Could you check a few things on this model? Use its own coordinates, in mm. Face numbers are marked on the shaded views. A direction names the side the tool comes from. Round coordinates to 2 decimals unless told otherwise and drop trailing zeros. Loops run counter-clockwise (first coordinate to the right, second up) from the corner with the lowest first, then second, coordinate; pieces in that order, holes last. Notation, with made-up numbers: M 16.5,54 L 49.5,54 A15 cw 49.5,63 Z; hole C 1.5,-30.5 d8. An arc over 180 degrees is marked long. Answer in a Markdown table with one row per item.
Autodesk Inventor part; units mm, degrees
ref_plane "YZ Plane" through (0, 0, 0) normal (1, 0, 0) x (0, 1, 0)
ref_plane "XZ Plane" through (0, 0, 0) normal (0, 1, 0) x (-1, 0, 0)
ref_plane "XY Plane" through (0, 0, 0) normal (0, 0, 1) x (1, 0, 0)
sketch "Sketch1" plane through (0, 0, 0) normal (0, 0, 1) x (1, 0, 0)
  line L0 (0, 0) -> (35, 0)
  line L1 (35, 0) -> (35, 82)
  line L2 (35, 82) -> (0, 82)
  line L3 (0, 82) -> (0, 0)
  line L4 (8.5, 79.95) -> (8.5, 77.05)
  line L5 (8.5, 77.05) -> (5.5, 77.05)
  line L6 (5.5, 77.05) -> (5.5, 53.95)
  line L7 (5.5, 33.6) -> (5.5, 6.85)
  line L8 (5.5, 6.85) -> (29.5, 6.85)
  line L9 (29.5, 6.85) -> (29.5, 79.95)
  line L10 (29.5, 79.95) -> (8.5, 79.95)
  line L11 (5.5, 53.95) -> (8.5, 53.95)
  line L12 (8.5, 53.95) -> (8.5, 33.6)
  line L13 (8.5, 33.6) -> (5.5, 33.6)
  circle A0 centre (19, 65.65) radius 2.25
  circle A1 centre (19, 21.45) radius 2.25
  dimension "d0" = 35
  dimension "d1" = 82
  dimension "d2" = 21
  dimension "d3" = 24
  dimension "d4" = 21
  dimension "d5" = 26.75
  dimension "d6" = 23.1
  dimension "d7" = 26
  dimension "d8" = 6.85
  dimension "d9" = 5.5
  dimension "d10" = 20.35
  dimension "d15" = 4.5
  dimension "d16" = 4.5
  dimension "d17" = 44.2
  dimension "d18" = 10.5
  dimension "d19" = 14.3
  dimension "d20" = 10.5
extrude "Extrusion1" add sketch "Sketch1" against normal blind 1.5 contours L10 L9 L8 L7 L13 L12 L11 L6 L5 L4 | A0 | A1
extrude "Extrusion3" add sketch "Sketch1" along normal blind 5 contours L3 L2 L1 L0 | L10 L9 L8 L7 L13 L12 L11 L6 L5 L4
sketch "Sketch2" plane through (0, 0, 5) normal (0, 0, 1) x (1, 0, 0)
  circle A0 centre (19, 21.45) radius 4.25
  circle A1 centre (19, 65.65) radius 4.25
  point P0 (0, 0)
  dimension "d23" = 8.5
  dimension "d24" = 8.5
extrude "Extrusion4" cut sketch "Sketch2" against normal blind 3
sketch "Sketch3" plane through (0, 0, 0) normal (0, -1, 0) x (1, 0, 0)
  line L0 (0, 5) -> (35, 5)
  line L1 (0, 0) -> (0, 5)
  line L2 (35, 0) -> (35, 5)
  line L3 (0, 5) -> (35, 5)
  line L4 (35, 5) -> (35, -32)
  line L5 (35, -32) -> (0, -32)
  line L6 (0, -32) -> (0, 5)
  line L7 (0, 0) -> (35, 0)
  line L8 (5.5, 0) -> (5.5, -1.5)
  line L9 (5.5, -8.5) -> (24.15, -8.5)
  line L10 (24.15, -8.5) -> (24.15, -11.35)
  line L11 (24.15, -11.35) -> (5.5, -11.35)
  line L12 (5.5, -11.35) -> (5.5, -8.5)
  dimension "d27" = 32
  dimension "d28" = 8.5
  dimension "d29" = 2.85
  dimension "d30" = 18.65
extrude "Extrusion5" add sketch "Sketch3" along normal blind 5 contours L0 L2 L7 L1 | L7 L4 L5 L6 | L9 L10 L11 L12
extrude "Extrusion6" add sketch "Sketch3" against normal blind 1.5 contours L9 L10 L11 L12
fillet "Fillet1" radius 1 1 edges at (29.5, 79.95, -0.75)
fillet "Fillet2" radius 1 1 edges at (8.5, 79.95, -0.75)
fillet "Fillet3" radius 1 1 edges at (5.5, 77.05, -0.75)
fillet "Fillet4" radius 1 1 edges at (5.5, 53.95, -0.75)
fillet "Fillet5" radius 1 1 edges at (5.5, 33.6, -0.75)
fillet "Fillet6" radius 1 1 edges at (5.5, 6.85, -0.75)
fillet "Fillet7" radius 1 1 edges at (29.5, 6.85, -0.75)
fillet "Fillet8" radius 1 1 edges at (5.5, 0.75, -11.35)
fillet "Fillet9" radius 1 3 edges at (24.15, 0.75, -11.35) (24.15, 0.75, -8.5) (5.5, 0.75, -8.5)
extrude "Extrusion7" cut sketch "Sketch1" against normal up to next contours A0 | A1
sketch "Sketch4" plane through (0, -5, 0) normal (0, -1, 0) x (1, 0, 0)
  line L0 (25.5, -24) -> (9.5, -24)
  line L1 (9.5, -24) -> (9.5, -8)
  line L2 (9.5, -8) -> (25.5, -8)
  line L3 (25.5, -8) -> (25.5, -24)
  line L4 (0, 5) -> (0, -32)
  line L5 (0, -32) -> (35, -32)
  point P0 (0, 0)
  dimension "d46" = 16
  dimension "d47" = 16
  dimension "d48" = 9.5
  dimension "d49" = 8
extrude "Extrusion8" add sketch "Sketch4" along normal blind 5
chamfer "Chamfer1" distance 5 angle 45 4 edges at (9.5, -5, -16) (17.5, -5, -24) (25.5, -5, -16) (17.5, -5, -8)
properties part number "keithley_2000_front_feet"
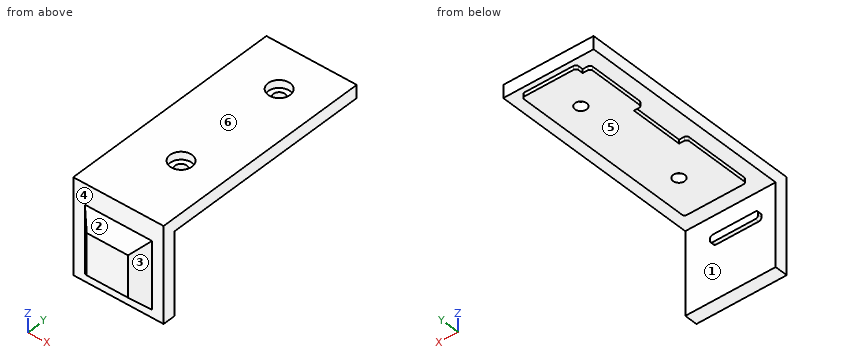
1) I want a section at D-D, the plane y = 47.5. Please give me the cut outline in (x, z), plus the area to 4 significant figures.
Computed:
| item | result |
|---|---|
| outline | M 0,0 L 8.5,0 L 8.5,-1.5 L 29.5,-1.5 L 29.5,0 L 35,0 L 35,5 L 0,5 Z |
| area | 206.5 mm² |
2) I want a section at B-B, the plane x = 19. State how many separate pieces and enclosed holes the cut face has, plus the area to 3 significant figures.
Computed:
| item | result |
|---|---|
| separate pieces | 3 |
| enclosed holes | 0 |
| area | 731 mm² |
3) If we mould it in two halves opening along Z, with no side actions, what happens to the marked faces 1, 2 and 3? For each: released by +Z, released by -Z, zero draft, split by the parting line, or undercut.
Computed:
| item | result |
|---|---|
| face 1 | undercut |
| face 2 | released by +Z |
| face 3 | zero draft |
4) Will these pins go through, and if not, where does the flat tip stop? P1, Ø5, axis at x = 26, y = 62, coming from the -Z side; P2, Ø0.8, axis at x = 17.5, y = 1, coming from the -Z side; P3, Ø1.2, axis at y = 23, z = -1, coming from the -X side.
Computed:
| item | result |
|---|---|
| P1 | stops at z = -1.5 |
| P2 | stops at z = -11.35 |
| P3 | stops at x = 5.5 |
5) Which directions (+Z, -Z, +X, -X, +Y, -Y) give clear straight access to the entire face, cutting with the end or side of a thin tool? Please do the marked faces 4, 5 and 6.
Computed:
| item | result |
|---|---|
| face 4 | -Y |
| face 5 | -Z, +X, -X, +Y |
| face 6 | +Z, +X, -X, +Y, -Y |
6) I want a section at A-A, the plane y = 21.45. Please give me the cut outline in (x, z).
Computed:
| item | result |
|---|---|
| outline | M 0,0 L 5.5,0 L 5.5,-1.5 L 16.75,-1.5 L 16.75,2 L 14.75,2 L 14.75,5 L 0,5 Z; M 21.25,-1.5 L 29.5,-1.5 L 29.5,0 L 35,0 L 35,5 L 23.25,5 L 23.25,2 L 21.25,2 Z |
7) I need wall thicknesses on line 1 (Y direction, x = 19, z = 0.2); line 2 (Y direction, x = 19, z = 4.15); line 3 (X direction, y = 21.45, z = -0.05). Which ranges of each line are inside material? Lowest first, please.
Computed:
| item | result |
|---|---|
| line 1 | y = -5 to 19.2, 23.7 to 63.4, 67.9 to 82 |
| line 2 | y = -5 to 17.2, 25.7 to 61.4, 69.9 to 82 |
| line 3 | x = 5.5 to 16.75, 21.25 to 29.5 |
